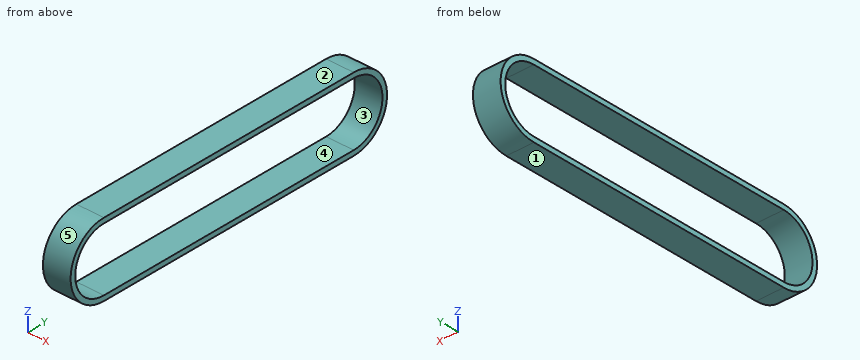
from build123d import *

# Parameters (mm, degrees)
F1_W = 6.35
F1_H = 1.15


with BuildPart() as f2:
    # F2: sweep along a path in F0
    with BuildLine(Plane.YZ) as f2_path:
        ThreePointArc((31.24, -7.7597), (38.9997, 0), (31.24, 7.7597))
        Line((31.24, 7.7597), (-31.24, 7.7597))
        ThreePointArc((-31.24, 7.7597), (-38.9997, 0), (-31.24, -7.7597))
        Line((-31.24, -7.7597), (31.24, -7.7597))
    # F1 (on Front) → F2 (sweep)
    with BuildSketch(Plane.XZ):
        with Locations((0, 7.7597)):
            Rectangle(F1_W, F1_H)
    sweep(path=f2_path.line)


solid = f2.part
Could you check a few things on this model? Use its own coordinates, in mm. Face numbers are marked on the shaded views. A direction names the side the tool comes from. Coordinates: 2 decimals unless noted, no trailing zeros. Order: outer loops, then holes, each group sorted by start corner. A loop starts at its lowest first (then second) coordinate and runs counter-clockwise, first axis right, second up. Notation, with made-up numbers: (34, 25) -> (85, 25) arc R17 cw to (85, 34) -> close; hole circle Ø7 at (16.5, -10.75). An arc over 180 degrees is marked (long way). One line per item, written item: value. Start each with the question number.
1) We'd pull the mould along Z, two halves only. Please class the marked faces 1, 2 and 3: +Z half, -Z half, draft (parallel to the pull), parting line (faces both ways), or undercut.
2) I'm going to push flat-ended pins straight in: pin 1 (2 mm diameter, centred on x = 0.5, z = -6, fed in from +Y); pin 2 (10 mm diameter, centred on y = -3, z = 1.5, fed in from +X). Where does each tip first touch, or does it pass through?
3) Imagine slicing it at A-A on z = 0. List the corners of the cut face in (x, y) for me (3 decimals), plus the area to 3 significant figures.
4) Imagine slicing it at C-C on x = 1. List the corners of the cut face in (y, z) for me, plus the area to 3 significant figures.
5) Imagine slicing it at B-B on y = 20.5. List the corners of the cut face in (x, z) for me (3 decimals), plus the area to 3 significant figures.
6) Which directions (+Z, -Z, +X, -X, +Y, -Y) give clear straight access to the entire face, cutting with the end or side of a thin tool? Please do the marked faces 4 and 5.
7) If I drill on L1, parallel to Z at x = -2.25, y = 29.5; L2, parallel to Y at x = 1.75, z = 6.25; L3, parallel to Y at x = -1.75, z = 2.75, over which ranges is the centre line in solid material (lowest first)? Write a range as [from, to].
Answer list:
1. face 1: -Z half
1. face 2: +Z half
1. face 3: undercut
2. pin 1: stops at y = 37.91
2. pin 2: passes through
3. outline: (-3.175, -39.575) -> (3.175, -39.575) -> (3.175, -38.425) -> (-3.175, -38.425) -> close; (-3.175, 38.425) -> (3.175, 38.425) -> (3.175, 39.575) -> (-3.175, 39.575) -> close
3. area: 14.6 mm2
4. outline: (-31.24, -8.33) -> (31.24, -8.33) arc R8.33 ccw to (31.24, 8.33) -> (-31.24, 8.33) arc R8.33 ccw to start; hole (-31.24, -7.18) -> (31.24, -7.18) arc R7.18 ccw to (31.24, 7.18) -> (-31.24, 7.18) arc R7.18 ccw to start
4. area: 200 mm2
5. outline: (-3.175, -8.335) -> (3.175, -8.335) -> (3.175, -7.185) -> (-3.175, -7.185) -> close; (-3.175, 7.185) -> (3.175, 7.185) -> (3.175, 8.335) -> (-3.175, 8.335) -> close
5. area: 14.6 mm2
6. face 4: +X, -X
6. face 5: +X, -X, -Y
7. L1: z = [-8.33, -7.18], [7.18, 8.33]
7. L2: y = [-36.75, -34.78], [34.78, 36.75]
7. L3: y = [-39.11, -37.88], [37.88, 39.11]
